Input: part model. Units: mm. Frame: model coordinates. Face numbers are marked on the shaded views. A direction names the side the tool comes from. Give positions to 0.01 mm unless a question says otherwise; leave off trailing zeros. Loops run counter-clockwise (first coordinate to the right, second up) from the corner with the lowest first, then second, coordinate; pieces in that order, holes last.
Autodesk Inventor part; units mm, degrees
ref_plane "YZ Plane" through (0, 0, 0) normal (1, 0, 0) x (0, 1, 0)
ref_plane "XZ Plane" through (0, 0, 0) normal (0, 1, 0) x (-1, 0, 0)
ref_plane "XY Plane" through (0, 0, 0) normal (0, 0, 1) x (1, 0, 0)
sketch "Sketch1" plane through (0, 0, 0) normal (1, 0, 0) x (0, 1, 0)
  line L0 (6.4158, 0) -> (3.2079, -5.5562)
  line L1 (3.2079, -5.5562) -> (-3.2079, -5.5562)
  line L2 (-3.2079, -5.5562) -> (-6.4158, 0)
  line L3 (-6.4158, 0) -> (-3.2079, 5.5563)
  line L4 (-3.2079, 5.5563) -> (3.2079, 5.5563)
  line L5 (3.2079, 5.5563) -> (6.4158, 0)
  point P0 (0, 0)
  point P1 (0, 0)
  dimension "d0" = 11.1125
extrude "Extrusion1" add sketch "Sketch1" along normal mid plane 4.9276
sketch "Sketch2" plane through (0, 0, 0) normal (0, 0, 1) x (1, 0, 0)
  line L0 (0, 0) -> (7.0752, 0)
  line L1 (-2.4638, 0) -> (-12.319, 0)
  line L2 (-2.4638, 0) -> (-2.4638, 4.7228)
  line L3 (-2.4638, 4.7228) -> (-2.9566, 4.7228)
  line L4 (-2.9566, 4.7228) -> (-2.9566, 5.1435)
  line L5 (-2.9566, 5.1435) -> (-12.319, 5.1435)
  line L6 (-12.319, 5.1435) -> (-12.319, 0)
  line L7 (-16.1978, 0) -> (10.954, 0)
  line L8 (-2.4638, 3.2079) -> (-2.4638, -3.2079)
  dimension "d3" = 9.8552
  dimension "d6" = 9.3624
  dimension "d32" = 10.287
  dimension "d33" = 9.4456
revolve "Revolution1" add sketch "Sketch2" angle 360 about axis through (-2.4638, 0, 0) along (-1, 0, 0)
mirror "Mirror1" about plane through (0, 0, 0) normal (1, 0, 0) of "Revolution1"
sketch "Sketch5" plane through (0, 0, 0) normal (0, 1, 0) x (-1, 0, 0)
  line L0 (2.4638, -5.5562) -> (-2.4638, -5.5562)
  line L1 (-2.4638, -5.5562) -> (-2.4638, -11.1125)
  line L2 (-2.4638, -5.5562) -> (0.1271, -11.1125)
  line L3 (-2.4638, -11.1125) -> (0.1271, -11.1125)
  line L4 (0, -12.2237) -> (0, -4.445)
  line L5 (3.4493, 0) -> (-3.4493, 0)
  dimension "d15" = 5.5563
  dimension "d38" = 25
revolve "Revolution4" cut sketch "Sketch5" angle 360 about axis through (-10, 0, 0) along (1, 0, 0) contours L2 L4 L3 L1 | L2 L3 L4
mirror "Mirror2" about plane through (0, 0, 0) normal (1, 0, 0) of "Revolution4"
chamfer "Chamfer1" distance 0.2223 angle 45 2 edges at (-12.319, -5.1435, 0) (12.319, -5.1435, 0)
hole "Hole1" at (-12.319, 0, 0) direction (1, 0, 0) diameter 5.588 end through all
thread "Rosca1"
thread "Thread2"
equation "\"d0\" = C_HEX"
equation "\"d1\" = 0.2 * L"
equation "\"d3\" = 0.4 * L"
equation "\"d6\" = 0.38 * L"
equation "\"d33\" = 0.85 * C_HEX"
equation "\"d17\" = 0.02 * C_HEX"
equation "\"d22\" = D"
equation "\"d15\" = 0.5 * C_HEX"
equation "\"C_HEX\" = 11.1125"
equation "\"L\" = 24.638"
equation "\"D\" = 5.588"
equation "\"ND1\" = 9.652"
equation "\"Parker_No\" = 1.2345"
properties part number "Boquilla hexagonal 216P de Parker 216P-2" material "Latón, amarillo claro"
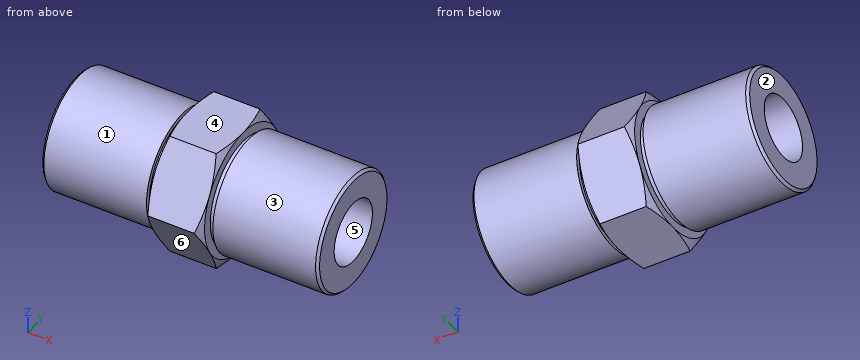
(1) Pin query (flat end, axial travel): pin 1 Ø1 at (x, z) = (-4, -3.5) entering from +Y; pin 2 Ø4 at (x, z) = (-8, -4.5) entering from +Y; pin 3 Ø6 at (x, y) = (7, 4.5) entering from -Z. Return the tip coordinate at first contact, or that it passes through.
Values follow:
pin 1: stops at y = 4.18
pin 2: stops at y = 4.5
pin 3: stops at z = -4.92
(2) Cut plane B-B (x = -7.5). Return the cut outline in (y, z), and give its area (3 significant figures).
Values follow:
outline: circle Ø10.29 at (0, 0); hole circle Ø5.59 at (0, 0)
area: 58.6 mm2
(3) Mould query, pull axis Y, two halves, no side actions, for the marked faces 4, 5 and 6. Classes: +Y half, -Y half, draft (parallel to the pull), parting line (faces both ways), or undercut.
Values follow:
face 4: draft
face 5: undercut
face 6: -Y half
(4) Reachability of the marked faces 1, 2 and 3 from +Z, -Z, +X, -X, +Y, -Y: full face, straight path, thin tool, end or side. Return the list, or none.
Values follow:
face 1: -X
face 2: +Z, -Z, -X, +Y, -Y
face 3: +X
(5) Ray query, probe 1 along Y at (x, z) = (-2.75, 0); probe 2 along Y at (x, z) = (4, 0); probe 3 along X at (y, z) = (2, -4.5). Return the intervals inside material, ascending.
Values follow:
probe 1: y = -4.72 to -2.79, 2.79 to 4.72
probe 2: y = -5.14 to -2.79, 2.79 to 5.14
probe 3: x = -12.32 to -2.96, -2.46 to 2.46, 2.96 to 12.32
(6) Cut plane A-A (x = 1.75). Return the cut outline in (y, z).
Values follow:
outline: (-6.42, 0) - (-3.21, -5.56) - (3.21, -5.56) - (6.42, 0) - (3.21, 5.56) - (-3.21, 5.56) - close; hole circle Ø5.59 at (0, 0)
